Read the model definition and answer for the solid it produces. Units are mm, in the model's axes. Face numbers are marked on the shaded views. A direction names the side the tool comes from. Give positions to 0.01 mm unless a question says otherwise; leave off trailing zeros. Order: outer loops, then holes, each group sorted by start corner. A loop starts at its lowest first (then second) coordinate and runs counter-clockwise, first axis right, second up. Notation, with made-up numbers: (32.25, -33) - (50.25, -33) arc R26 ccw to (50.25, 6) - close; hole circle Ø1 at (38.5, 36.5). An arc over 180 degrees is marked (long way). Return JSON: item names as keys, results as strings.
```python
from build123d import *

# Parameters (mm, degrees)
CROQUIS1_W              = 20
CROQUIS1_H              = 20
SALIENTE_EXTRUIR1_DEPTH = 2
CROQUIS2_R              = 3.395302969
CROQUIS2_R_2            = 4.300626918
CROQUIS2_W              = 3.832057349
CROQUIS2_H              = 4.474113334
SALIENTE_EXTRUIR2_DEPTH = 7
CROQUIS3_R              = 1.048920166
CORTAR_EXTRUIR1_DEPTH   = 2


with BuildPart() as part:
    # Croquis1 → Saliente-Extruir1 (new body)
    with BuildSketch(Plane.XY):
        Rectangle(CROQUIS1_W, CROQUIS1_H)
    extrude(amount=SALIENTE_EXTRUIR1_DEPTH)

    # Croquis2 → Saliente-Extruir2 (add)
    with BuildSketch(Plane.XY.offset(2)):
        with Locations(Location((0, 5.24700562, 0), (0, 0, 180))):
            Circle(CROQUIS2_R)
        with Locations(Location((0, -3.577988987, 0), (0, 0, 180))):
            Circle(CROQUIS2_R_2)
        with Locations((-7.217868445, 3.658804494)):
            Rectangle(CROQUIS2_W, CROQUIS2_H)
    extrude(amount=SALIENTE_EXTRUIR2_DEPTH)

    # Croquis3 → Cortar-Extruir1 (cut)
    with BuildSketch(Plane.XY.offset(2)):
        with Locations((8.280127459, 4.598002093)):
            Circle(CROQUIS3_R)
        with Locations((8.280127459, 1.598002093)):
            Circle(CROQUIS3_R)
        with Locations((8.280127459, -1.401997907)):
            Circle(CROQUIS3_R)
        with Locations((8.280127459, -4.401997907)):
            Circle(CROQUIS3_R)
    extrude(amount=-CORTAR_EXTRUIR1_DEPTH, mode=Mode.SUBTRACT)


solid = part.part
```
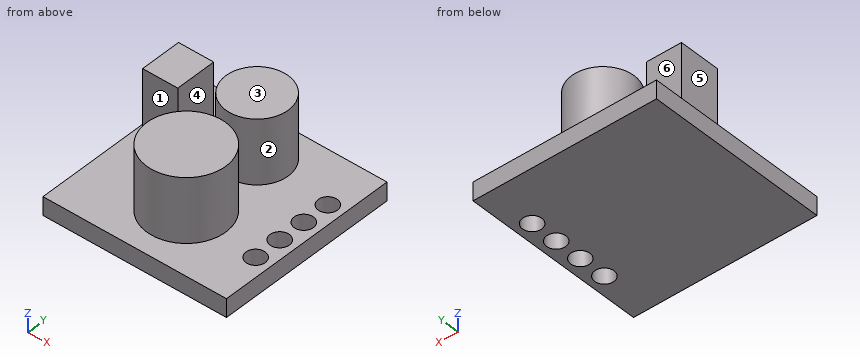
Q1. Given pin 1 (1.5 mm diameter, centred on x = 0.5, z = 3, fed in from +Y); pin 2 (2.5 mm diameter, centred on x = 8.28, y = -1.4, fed in from +Z); pin 3 (5 mm diameter, centred on x = 3.5, z = 6, fed in from -Y), each flat-ended and moving along its own axis, determine where each tip first touches the part or whether it passes through.
Values:
{"pin 1": "stops at y = 8.64", "pin 2": "stops at z = 2", "pin 3": "stops at y = -7.76"}
Q2. A cutting plane is placed at A-A (z = 3.75). Write down the section's boundary in (x, y).
Values:
{"outline": "(-9.13, 1.42) - (-5.3, 1.42) - (-5.3, 5.9) - (-9.13, 5.9) - close; circle Ø8.6 at (0, -3.58); circle Ø6.79 at (0, 5.25)"}
Q3. For the marked faces 4, 5 and 6, determine the directions among +Z, -Z, +X, -X, +Y, -Y from which every point of the face is accessible in a straight line to the end or side of a thin tool.
Values:
{"face 4": "+Z, +Y, -Y", "face 5": "+Z, -X, +Y, -Y", "face 6": "+Z, -X, +Y"}
Q4. Determine the mould class of the marked faces 1, 2 and 3 for opening direction Y: released by +Y, released by -Y, zero draft, split by the parting line, or undercut.
Values:
{"face 1": "released by -Y", "face 2": "undercut", "face 3": "zero draft"}
Q5. A cutting plane is placed at B-B (x = 0). Write down the section's boundary in (y, z), and give its area (3 significant figures).
Values:
{"outline": "(-10, 0) - (10, 0) - (10, 2) - (8.64, 2) - (8.64, 9) - (1.85, 9) - (1.85, 2) - (0.72, 2) - (0.72, 9) - (-7.88, 9) - (-7.88, 2) - (-10, 2) - close", "area": "148 mm²"}
Q6. A cutting plane is placed at C-C (z = 1.25). Write down the section's boundary in (x, y).
Values:
{"outline": "(-10, -10) - (10, -10) - (10, 10) - (-10, 10) - close; hole circle Ø2.1 at (8.28, -4.4); hole circle Ø2.1 at (8.28, -1.4); hole circle Ø2.1 at (8.28, 1.6); hole circle Ø2.1 at (8.28, 4.6)"}
Q7. Consider L1, parallel to Y at x = 7.5, z = 0.5; L2, parallel to Z at x = -5.5, y = 6.25; L3, parallel to Y at x = -8.25, z = 2.75. Determine where each line is inside the solid, lowest interval first.
Values:
{"L1": "y = -10 to -5.1, -3.7 to -2.1, -0.7 to 0.9, 2.3 to 3.9, 5.3 to 10", "L2": "z = 0 to 2", "L3": "y = 1.42 to 5.9"}
Q8. A cutting plane is placed at D-D (y = 0.25). Write down the section's boundary in (x, z).
Values:
{"outline": "(-10, 0) - (10, 0) - (10, 2) - (1.96, 2) - (1.96, 9) - (-1.96, 9) - (-1.96, 2) - (-10, 2) - close"}
